The figure shows three views and two pictorial views of one solid part (mm, origin at its lowest corner). Answer the questions. Give positions to 0.01 mm unless a question says otherwise; leave off trailing zeros. Loops run counter-clockwise (first coordinate to the right, second up) from the corner with the lowest first, then second, coordinate; pieces in that order, holes last. Notation, with made-up numbers: M -24.5,-26 L 18.5,-26 A15 ccw 18.5,-14 Z; hole C 72,-16.75 d3. An arc over 180 degrees is marked long. Write item = value, one per line. Start each with the question number.
1. Consider L1, parallel to Y at x = 4, z = 1.05; L2, parallel to Y at x = 2.75, z = 3.6; L3, parallel to X at y = 3, z = 1.6. Determine where each line is inside the solid, lowest interval first. Write a range as [from, to].
2. Section C-C on z = 3.2 is taken. Determine the outline of the cut face in (x, y), plus the area to 3 significant figures.
3. Section A-A on x = 4 is taken. Determine the outline of the cut face in (y, z).
4. The mould has two halves that part along Y. Classify the marked faces 1, 2, 3 and 4: released by +Y, released by -Y, zero draft, split by the parting line, or undercut.
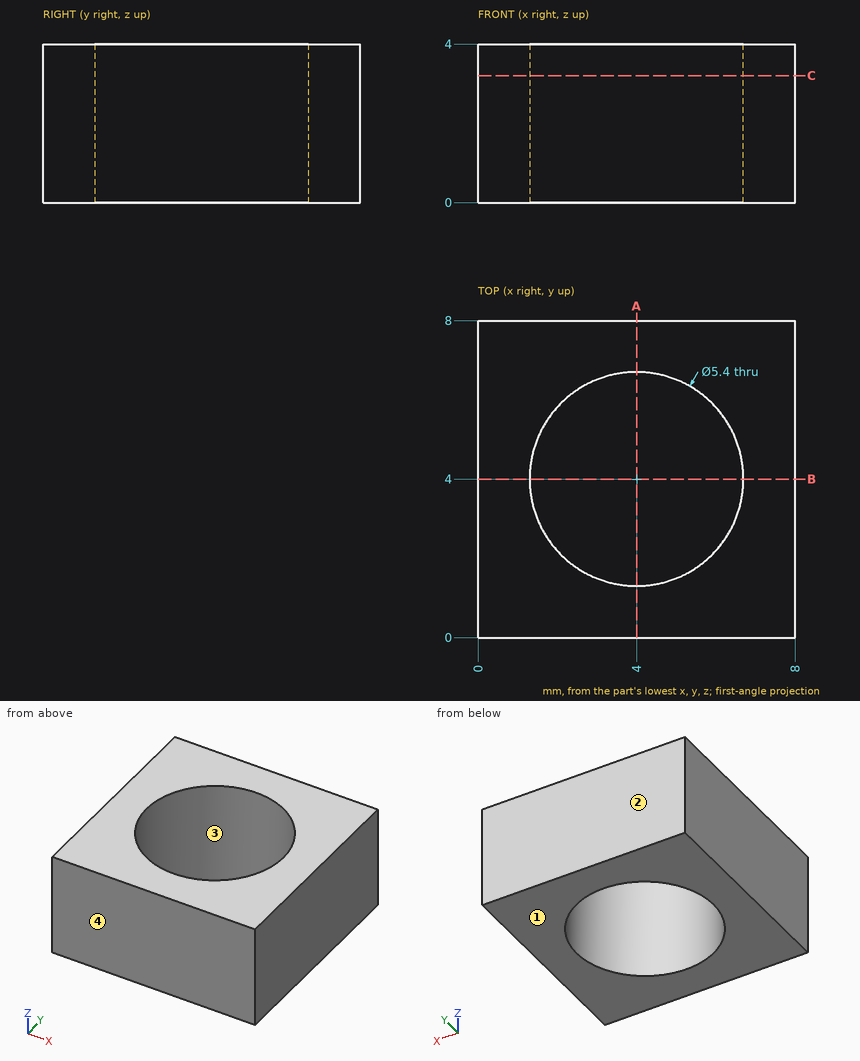
Verdict:
q1.L1 = [0, 1.3], [6.7, 8]
q1.L2 = [0, 1.61], [6.39, 8]
q1.L3 = [0, 1.49], [6.51, 8]
q2.outline = M 0,0 L 8,0 L 8,8 L 0,8 Z; hole C 4,4 d5.4
q2.area = 41.1 mm2
q3.outline = M 0,0 L 1.3,0 L 1.3,4 L 0,4 Z; M 6.7,0 L 8,0 L 8,4 L 6.7,4 Z
q4.face_1 = zero draft
q4.face_2 = released by +Y
q4.face_3 = undercut
q4.face_4 = released by -Y
